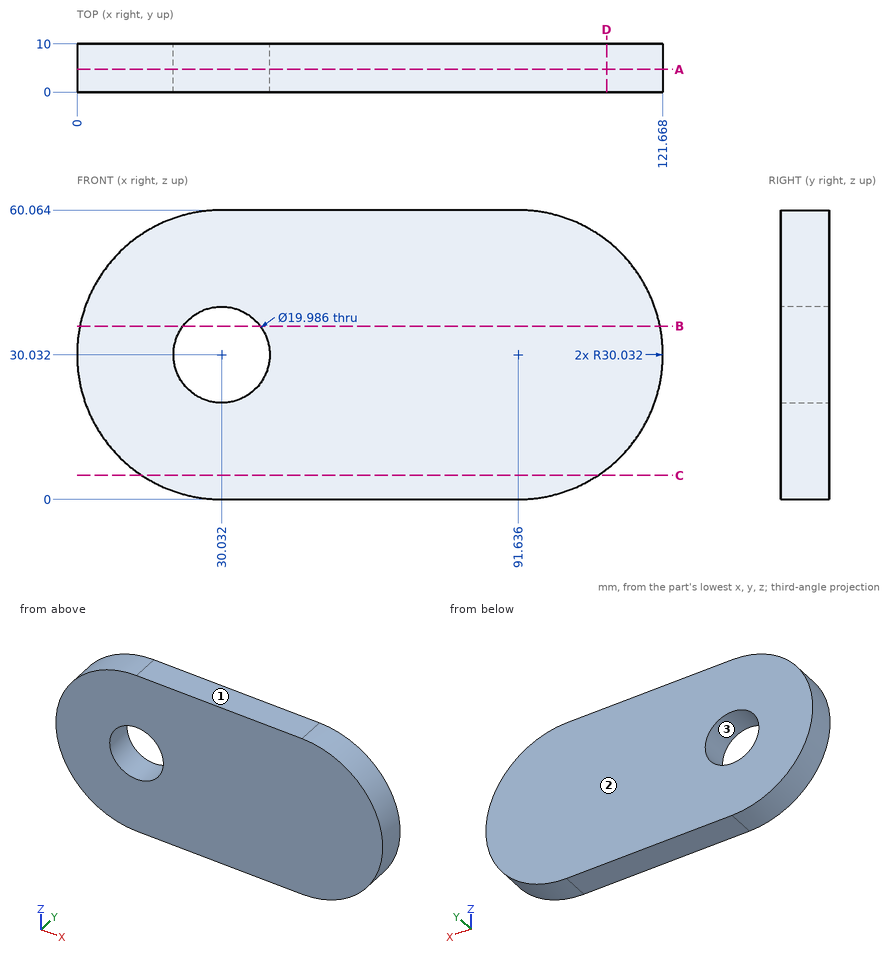
Verification items for this drawing (mm, ordinates from the low corner). Give positions to 0.01 mm unless a question says otherwise; leave off trailing zeros. Loops run counter-clockwise (first coordinate to the right, second up) from the corner with the lowest first, then second, coordinate; pieces in that order, holes last. Notation, with made-up numbers: M -32,-28.5 L 23,-28.5 A30 ccw 23,-6.5 Z; hole C 32.5,-18 d5. An arc over 180 degrees is marked long. Write item = value, one per line. Start each with the question number.
1. Go/stop test with flat-tipped pins: P1, Ø6, axis at y = 1.5, z = 52, coming from the +X side; P2, Ø1, axis at x = 46, y = 8.5, coming from the -Z side; P3, Ø2, axis at y = 5.5, z = 40, coming from the +X side. Record where each tip stops, or that it passes through.
2. Thickness scan on probe 1 along Z at (x, y) = (26, 2.25) (1 decimal); probe 2 along Z at (x, y) = (92.5, 7.75); probe 3 along X at (y, z) = (7, 22) (1 decimal). Record the ranges inside material, lowest first.
3. Section check D-D, the plane x = 110. Enter the section's corners in (y, z) (1 decimal).
4. Section check C-C, the plane z = 5. Enter the section's corners in (x, y), plus the area to 3 significant figures.
5. Section check B-B, the plane z = 36. Enter the section's corners in (x, y).
6. Draft check along Z on the marked faces 1, 2 and 3. Enter one of: +Z half, -Z half, draft (parallel to the pull), parting line (faces both ways), or undercut.
7. Section check A-A, the plane y = 4.75. Enter the section's corners in (x, z) (1 decimal).
Values follow:
q1.P1 = 114.92
q1.P2 = 0
q1.P3 = 120.3
q2.probe_1 = 0.3 to 20.9, 39.2 to 59.8
q2.probe_2 = 0.01 to 60.05
q2.probe_3 = 1.1 to 24.1, 36 to 120.6
q3.outline = M 0,6.3 L 10,6.3 L 10,53.8 L 0,53.8 Z
q4.outline = M 13.44,0 L 108.23,0 L 108.23,10 L 13.44,10 Z
q4.area = 948 mm^2
q5.outline = M 0.6,0 L 22.02,0 L 22.02,10 L 0.6,10 Z; M 38.05,0 L 121.07,0 L 121.07,10 L 38.05,10 Z
q6.face_1 = +Z half
q6.face_2 = draft
q6.face_3 = undercut
q7.outline = M 30,0 L 91.6,0 A30 ccw 91.6,60.1 L 30,60.1 A30 ccw Z; hole C 30,30 d20
